Here's how the part is built. I have some questions about the finished solid (model axes, mm). Face numbers are marked on the shaded views. A direction names the side the tool comes from. Coordinates: 2 decimals unless noted, no trailing zeros. Write each loop counter-clockwise with the first axis right and the second up, starting at its lowest first coordinate (ties: lowest second). Pieces come first, ordered by that corner, then holes. Notation, with made-up numbers: M -30.75,10 L -3.75,10 A25 ccw -3.75,31 Z; hole C 20.25,81.5 d1. An arc over 180 degrees is marked long. Use a Markdown table: item, result.
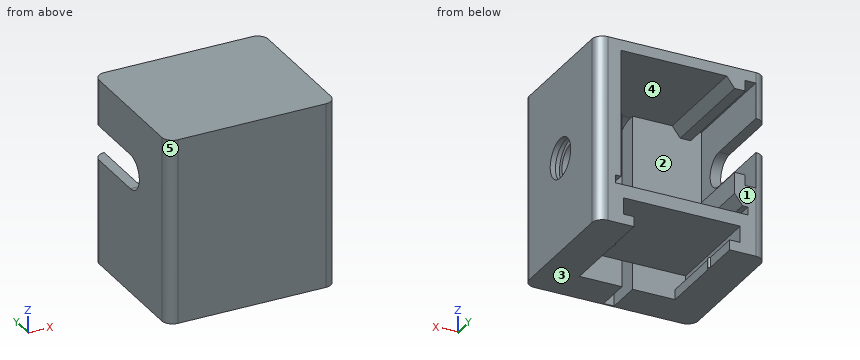
```python
from build123d import *

# Parameters (mm, degrees)
SKETCH1_W               = 32
SKETCH1_H               = 27
BOSS_EXTRUDE1_DEPTH     = 35
FILLET1_R               = 2
CUT_EXTRUDE1_DEPTH      = 1
CUT_EXTRUDE1_DEPTH_BACK = 28
BOSS_EXTRUDE2_DEPTH     = 7
BOSS_EXTRUDE3_DEPTH     = 1.9
SKETCH5_W               = 2
SKETCH5_H               = 7
CUT_EXTRUDE2_DEPTH      = 33
CUT_EXTRUDE3_DEPTH      = 20
SKETCH7_W               = 2
SKETCH7_H               = 33
BOSS_EXTRUDE4_DEPTH     = 0.25
FILLET2_R               = 6
CUT_EXTRUDE5_DEPTH      = 4.5
SKETCH14_W              = 2.5
SKETCH14_H              = 20
CUT_EXTRUDE6_DEPTH      = 20
SKETCH16_W              = 2
SKETCH16_H              = 4
SKETCH16_H_2            = 2
BOSS_EXTRUDE5_DEPTH     = 20
BOSS_EXTRUDE6_DEPTH     = 20


with BuildPart() as part:
    # Sketch1 → Boss-Extrude1 (new body)
    with BuildSketch(Plane.XY):
        Rectangle(SKETCH1_W, SKETCH1_H)
    extrude(amount=BOSS_EXTRUDE1_DEPTH)

    # Fillet1
    fillet1_edges = [part.edges().sort_by_distance(p)[0] for p in [
        (16, -13.5, 17.5),
        (-16, -13.5, 17.5),
        (-16, 13.5, 17.5),
        (16, 13.5, 17.5),
    ]]
    fillet(fillet1_edges, radius=FILLET1_R)

    # Sketch2 → Cut-Extrude1 (cut, two sides)
    with BuildSketch(Plane.XZ.offset(13.5)) as cut_extrude1_sk:
        Polygon((-9.05, 0), (-9.05, 1.9), (-11.05, 1.9), (-11.05, 5), (11.05, 5), (11.05, 1.9), (9.05, 1.9), (9.05, 0), align=None)
    extrude(amount=CUT_EXTRUDE1_DEPTH, mode=Mode.SUBTRACT)
    extrude(cut_extrude1_sk.sketch, amount=-CUT_EXTRUDE1_DEPTH_BACK, mode=Mode.SUBTRACT)

    # Sketch3 → Boss-Extrude2 (add)
    with BuildSketch(Plane.XZ.offset(13.5)):
        Polygon((-9.05, 0), (-9.05, 1.9), (-11.05, 1.9), (-11.05, 5), (11.05, 5), (11.05, 1.9), (9.05, 1.9), (9.05, 0), align=None)
    extrude(amount=-BOSS_EXTRUDE2_DEPTH)

    # Sketch4 → Boss-Extrude3 (add)
    with BuildSketch(Plane(origin=(0, 0, 1.9), x_dir=(-1, 0, 0), z_dir=(0, 0, -1))):
        with BuildLine():
            Line((-9.05, 6.5), (-9.05, 5.5))
            ThreePointArc((-9.05, 5.5), (-8.8, 6), (-9.05, 6.5))
        make_face()
    boss_extrude3 = extrude(amount=BOSS_EXTRUDE3_DEPTH)

    # Mirror1: Boss-Extrude3 across plane
    add(boss_extrude3.mirror(Plane(origin=(0, 0, 0), x_dir=(0, 0, 1), z_dir=(1, 0, 0))))

    # Sketch5 → Cut-Extrude2 (cut)
    with BuildSketch(Plane(origin=(0, 0, 0), x_dir=(-1, 0, 0), z_dir=(0, 0, -1))):
        with Locations((0, -10)):
            Rectangle(SKETCH5_W, SKETCH5_H)
    extrude(amount=-CUT_EXTRUDE2_DEPTH, mode=Mode.SUBTRACT)

    # Sketch6 → Cut-Extrude3 (cut)
    with BuildSketch(Plane(origin=(0, 13.5, 0), x_dir=(1, 0, 0), z_dir=(0, 1, 0))):
        Polygon((-12.5, -7.5), (-12.5, -9), (-11.5, -9), (-11.5, -33), (11.5, -33), (11.5, -9), (12.5, -9), (12.5, -7.5), align=None)
    extrude(amount=-CUT_EXTRUDE3_DEPTH, mode=Mode.SUBTRACT)

    # Sketch7 → Boss-Extrude4 (add)
    with BuildSketch(Plane.XZ.offset(13.5)):
        with Locations((0, 16.5)):
            Rectangle(SKETCH7_W, SKETCH7_H)
    extrude(amount=-BOSS_EXTRUDE4_DEPTH)

    # Fillet2
    fillet2_edges = [part.edges().sort_by_distance(p)[0] for p in [
        (0, -13.25, 33),
    ]]
    fillet(fillet2_edges, radius=FILLET2_R)

    # Sketch9 → Cut-Revolve1 (revolve, cut)
    with BuildSketch(Plane(origin=(0, 0, 17.75), x_dir=(-1, 0, 0), z_dir=(0, 0, -1))):
        Polygon((-15, 4.25), (-14, 4.25), (-14, 3.325), (-11.5, 3.325), (-11.5, 0), (-16, 0), (-16, 3.75), (-15, 3.75), align=None)
    revolve(axis=Axis((16, 0, 17.75), (-1, 0, 0)), mode=Mode.SUBTRACT)

    # Sketch11 → Cut-Extrude5 (cut)
    with BuildSketch(Plane(origin=(-16, 0, 44), x_dir=(0, 0, -1), z_dir=(1, 0, 0))):
        with BuildLine():
            Line((24.25, 23), (24.25, 0))
            ThreePointArc((24.25, 0), (21, -3.25), (17.75, 0))
            Line((17.75, 0), (17.75, 23))
            ThreePointArc((17.75, 23), (21, 26.25), (24.25, 23))
        make_face()
    extrude(amount=CUT_EXTRUDE5_DEPTH, mode=Mode.SUBTRACT)

    # Sketch14 → Cut-Extrude6 (cut)
    with BuildSketch(Plane(origin=(0, 13.5, 0), x_dir=(1, 0, 0), z_dir=(0, 1, 0))):
        with Locations((-12.75, -23)):
            Rectangle(SKETCH14_W, SKETCH14_H)
    extrude(amount=-CUT_EXTRUDE6_DEPTH, mode=Mode.SUBTRACT)

    # Sketch16 → Boss-Extrude5 (add)
    with BuildSketch(Plane(origin=(0, 13.5, 0), x_dir=(1, 0, 0), z_dir=(0, 1, 0))):
        with Locations((-11, -13)):
            Rectangle(SKETCH16_W, SKETCH16_H)
        with Locations((-11, -32)):
            Rectangle(SKETCH16_W, SKETCH16_H_2)
    extrude(amount=-BOSS_EXTRUDE5_DEPTH)

    # Sketch20 → Boss-Extrude6 (add)
    with BuildSketch(Plane(origin=(0, 13.5, 0), x_dir=(1, 0, 0), z_dir=(0, 1, 0))):
        Polygon((-11.5, -9), (-10, -11), (-11.5, -11), align=None)
        Polygon((-10, -31), (-8.5, -33), (-10, -33), align=None)
    extrude(amount=-BOSS_EXTRUDE6_DEPTH)


solid = part.part
```
1. Which directions (+Z, -Z, +X, -X, +Y, -Y) give clear straight access to the entire face, cutting with the end or side of a thin tool? Please do the marked faces 4 and 5.
Answers follow:
| item | result |
|---|---|
| face 4 | +Y |
| face 5 | +Z, -Z, -X, -Y |
2. Suppose I cut it at C-C on z = 23. Write out the boundary of the cut face in (x, y), and give its area (3 significant figures).
Answers follow:
| item | result |
|---|---|
| outline | M -16,-11.5 A2 ccw -14,-13.5 L 14,-13.5 A2 ccw 16,-11.5 L 16,11.5 A2 ccw 14,13.5 L 11.5,13.5 L 11.5,-6.5 L 1,-6.5 L 1,-13.25 L -1,-13.25 L -1,-6.5 L -14,-6.5 L -14,-3.25 L -16,-3.25 Z |
| area | 304 mm2 |
3. Suppose I cut it at B-B on x = -4. Write out the boundary of the cut face in (y, z), and give its area (3 significant figures).
Answers follow:
| item | result |
|---|---|
| outline | M -13.5,0 L -6.5,0 L -6.5,5 L 13.5,5 L 13.5,7.5 L -6.5,7.5 L -6.5,33 L 13.5,33 L 13.5,35 L -13.5,35 Z |
| area | 335 mm2 |
4. We'd pull the mould along Z, two halves only. Please class the marked faces 1, 2 and 3: +Z half, -Z half, draft (parallel to the pull), parting line (faces both ways), or undercut.
Answers follow:
| item | result |
|---|---|
| face 1 | draft |
| face 2 | undercut |
| face 3 | -Z half |
5. Suppose I cut it at A-A on z = 17.75. Write out the boundary of the cut face in (x, y) (3 decimals), and give its area (3 significant figures).
Answers follow:
| item | result |
|---|---|
| outline | M -16,-11.5 A2 ccw -14,-13.5 L 14,-13.5 A2 ccw 16,-11.5 L 16,-3.75 L 15,-3.75 L 15,-4.25 L 14,-4.25 L 14,-3.325 L 11.5,-3.325 L 11.5,-6.5 L 1,-6.5 L 1,-13.25 L -1,-13.25 L -1,-6.5 L -14,-6.5 L -14,13.5 A2 ccw -16,11.5 Z; M 11.5,3.325 L 14,3.325 L 14,4.25 L 15,4.25 L 15,3.75 L 16,3.75 L 16,11.5 A2 ccw 14,13.5 L 11.5,13.5 Z |
| area | 304 mm2 |
6. Will these pins go through, and if not, where does the flat tip stop? pin 1 Ø6 at (y, z) = (0, 17.75) entering from +X; pin 2 Ø2.5 at (y, z) = (0, 16.5) entering from +X; pin 3 Ø4 at (x, z) = (-7.5, 16.5) entering from +Y.
Answers follow:
| item | result |
|---|---|
| pin 1 | stops at x = -10 |
| pin 2 | stops at x = -14 |
| pin 3 | stops at y = -6.5 |
7. I need wall thicknesses on probe 1 along Z at (x, y) = (12.1, 0) (3 decimals); probe 2 along X at (y, z) = (10.75, 14); probe 3 along Z at (x, y) = (-5, 9.25). Which ranges of each line are inside material? Lowest first, please.
Answers follow:
| item | result |
|---|---|
| probe 1 | z = 0 to 7.5, 9 to 14.425, 21.075 to 35 |
| probe 2 | x = -16 to -14, -12 to -10, 11.5 to 16 |
| probe 3 | z = 5 to 7.5, 33 to 35 |
